Could you check a few things on this model? Use its own coordinates, in mm. Round coordinates to 2 decimals unless told otherwise and drop trailing zeros. Loops run counter-clockwise (first coordinate to the right, second up) from the corner with the lowest first, then second, coordinate; pieces in that order, holes last. Notation, with made-up numbers: M -13,43 L 36,43 A17 cw 36,57 Z; hole C 41,-15 d5. An arc over 180 degrees is marked long. Return JSON: item names as keys, results as strings. Group by question number.
```python
from build123d import *

# Parameters (mm, degrees)
SKETCH_1_W                = 45
SKETCH_1_H                = 45
EXTRUDE_1_DEPTH           = 4
SKETCH_2_R                = 1.525
CUT_EXTRUDE_1_DEPTH       = 4
FILLET_1_R                = 3
HOLE_WIZARD_1_D           = 3
HOLE_WIZARD_1_CSINK_D     = 6
HOLE_WIZARD_1_CSINK_ANGLE = 90
SKETCH_5_R                = 1.525
CUT_EXTRUDE_2_DEPTH       = 10
HOLE_WIZARD_2_D           = 3
HOLE_WIZARD_2_CSINK_D     = 6
HOLE_WIZARD_2_CSINK_ANGLE = 90
CUT_EXTRUDE_3_DEPTH       = 1
CUT_EXTRUDE_3_DEPTH_BACK  = 5
FILLET_2_R                = 2
SKETCH_3_R                = 1.525
CUT_EXTRUDE_4_DEPTH       = 1
CUT_EXTRUDE_4_DEPTH_BACK  = 5


with BuildPart() as part:
    # 草图1 → 凸台-拉伸1 (new body)
    with BuildSketch(Plane(origin=(0, 0, 0), x_dir=(1, 0, 0), z_dir=(0, 1, 0))):
        Rectangle(SKETCH_1_W, SKETCH_1_H)
    extrude(amount=EXTRUDE_1_DEPTH)

    # 草图2 → 切除-拉伸1 (cut)
    with BuildSketch(Plane(origin=(0, 4, 0), x_dir=(1, 0, 0), z_dir=(0, 1, 0))):
        with Locations((-19, 0)):
            Circle(SKETCH_2_R)
        with Locations((19, 0)):
            Circle(SKETCH_2_R)
    extrude(amount=-CUT_EXTRUDE_1_DEPTH, mode=Mode.SUBTRACT)

    # 圆角1
    fillet_1_edges = [part.edges().sort_by_distance(p)[0] for p in [
        (22.5, 2, 22.5),
        (-22.5, 2, 22.5),
        (-22.5, 2, -22.5),
        (22.5, 2, -22.5),
    ]]
    fillet(fillet_1_edges, radius=FILLET_1_R)

    # 孔1 (through all)
    with Locations(Plane(origin=(-15, 4, -19.75), x_dir=(0, 0, 1), z_dir=(0, 1, 0))):
        with Locations((0, 0), (0, 20)):
            CounterSinkHole(HOLE_WIZARD_1_D / 2, HOLE_WIZARD_1_CSINK_D / 2, counter_sink_angle=HOLE_WIZARD_1_CSINK_ANGLE)

    # 草图5 → 切除-拉伸2 (cut)
    with BuildSketch(Plane(origin=(0, 4, 0), x_dir=(1, 0, 0), z_dir=(0, 1, 0))):
        with Locations((0, 19)):
            Circle(SKETCH_5_R)
        with Locations((0, -19)):
            Circle(SKETCH_5_R)
    extrude(amount=-CUT_EXTRUDE_2_DEPTH, mode=Mode.SUBTRACT)

    # 孔2 (through all)
    with Locations(Plane(origin=(0, 0, 0), x_dir=(-1, 0, 0), z_dir=(0, -1, 0))):
        with Locations((0, 19)):
            CounterSinkHole(HOLE_WIZARD_2_D / 2, HOLE_WIZARD_2_CSINK_D / 2, counter_sink_angle=HOLE_WIZARD_2_CSINK_ANGLE)

    # 草图8 → 切除-拉伸3 (cut, two sides)
    with BuildSketch(Plane(origin=(0, 4, 0), x_dir=(1, 0, 0), z_dir=(0, 1, 0))) as cut_extrude_3_sk:
        Polygon((0, 10.606601718), (-10.606601718, 0), (0, -10.606601718), (10.606601718, 0), align=None)
    extrude(amount=CUT_EXTRUDE_3_DEPTH, mode=Mode.SUBTRACT)
    extrude(cut_extrude_3_sk.sketch, amount=-CUT_EXTRUDE_3_DEPTH_BACK, mode=Mode.SUBTRACT)

    # 圆角2
    fillet_2_edges = [part.edges().sort_by_distance(p)[0] for p in [
        (0, 2, -10.606601718),
        (10.606601718, 2, 0),
        (0, 2, 10.606601718),
        (-10.606601718, 2, 0),
    ]]
    fillet(fillet_2_edges, radius=FILLET_2_R)

    # 草图3 → 切除-拉伸4 (cut, two sides)
    with BuildSketch(Plane(origin=(0, 4, 0), x_dir=(1, 0, 0), z_dir=(0, 1, 0))) as cut_extrude_4_sk:
        with Locations((5, 19.75)):
            Circle(SKETCH_3_R)
        with Locations((-15, 19.75)):
            Circle(SKETCH_3_R)
    extrude(amount=CUT_EXTRUDE_4_DEPTH, mode=Mode.SUBTRACT)
    extrude(cut_extrude_4_sk.sketch, amount=-CUT_EXTRUDE_4_DEPTH_BACK, mode=Mode.SUBTRACT)


solid = part.part
```
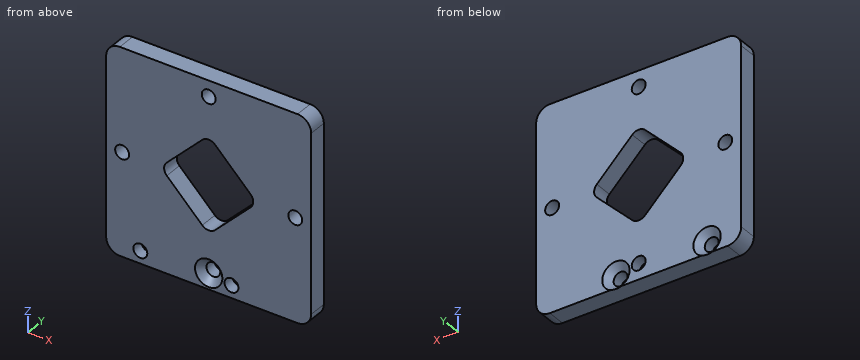
1. I'm going to push a flat-ended pin straight in: pin 1 Ø3.5 at (x, z) = (5, -19.75) entering from -Y. Where does the tip first touch, or does it pass through?
2. If we section it at D-D, the plane z = -6.5: Please give me the cut outline in (x, y), then the cut area to 3 significant figures.
3. If we section it at A-A, the plane x = -15: Please give me the cut outline in (y, z) (3 decimals).
4. If we section it at B-B, the plane y = 3.1: Please give me the cut outline in (x, z) (3 decimals), then the cut area to 3 significant figures.
5. I need wall thicknesses on probe 1 along Z at (x, y) = (0, 2.65) (3 decimals); probe 2 along X at (y, z) = (1, 19) (3 decimals). Which ranges of each line are inside material? Lowest first, please.
6. If we section it at C-C, the plane x = 0: Please give me the cut outline in (y, z) (3 decimals), then the cut area to 3 significant figures.
Geometry results:
{
 "1": {"pin 1": "y = 0"},
 "2": {"outline": "M -22.5,0 L -4.11,0 L -4.11,4 L -22.5,4 Z; M 4.11,0 L 22.5,0 L 22.5,4 L 4.11,4 Z", "area": "147 mm^2"},
 "3": {"outline": "M 0,-22.5 L 3.75,-22.5 L 2.525,-21.275 L 0,-21.275 Z; M 0,-18.225 L 2.525,-18.225 L 4,-16.75 L 4,22.5 L 0,22.5 Z"},
 "4": {"outline": "M -22.5,-19.5 A3 ccw -19.5,-22.5 L 19.5,-22.5 A3 ccw 22.5,-19.5 L 22.5,19.5 A3 ccw 19.5,22.5 L -19.5,22.5 A3 ccw -22.5,19.5 Z; hole C -19,0 d3.05; hole C -15,-19.75 d4.2; hole M -9.192,-1.414 L -1.414,-9.192 A2 ccw 1.414,-9.192 L 9.192,-1.414 A2 ccw 9.192,1.414 L 1.414,9.192 A2 ccw -1.414,9.192 L -9.192,1.414 A2 ccw Z; hole C 0,-19 d3.05; hole C 0,19 d3.05; hole C 5,-19.75 d4.2; hole C 19,0 d3.05", "area": "1,740 mm^2"},
 "5": {"probe 1": "-22.5 to -20.525, -17.475 to -9.778, 9.778 to 17.475, 20.525 to 22.5", "probe 2": "-22.5 to -1.525, 1.525 to 22.5"},
 "6": {"outline": "M 0,-22.5 L 4,-22.5 L 4,-20.525 L 1.475,-20.525 L 0,-22 Z; M 0,-16 L 1.475,-17.475 L 4,-17.475 L 4,-9.778 L 0,-9.778 Z; M 0,9.778 L 4,9.778 L 4,17.475 L 0,17.475 Z; M 0,20.525 L 4,20.525 L 4,22.5 L 0,22.5 Z", "area": "75.2 mm^2"}
}
